from build123d import *

# Parameters (mm, degrees)
F0_R     = 42.5
F0_R_2   = 27.5
F1_DEPTH = 33.5
F2_R     = 100
F2_R_2   = 42.5
F2_R_3   = 27.5
F3_DEPTH = 4
F4_R     = 100
F4_R_2   = 42.5
F4_R_3   = 27.5
F5_DEPTH = 4


# Not quite as in the source:
# - a feature names something its author has since deleted; it is built from what else it names


with BuildPart() as f1:
    # F0 (on Right) → F1 (new body, symmetric)
    with BuildSketch(Plane.YZ):
        Circle(F0_R)
        Circle(F0_R_2, mode=Mode.SUBTRACT)
    extrude(amount=F1_DEPTH, both=True)

    # F2 (on face) → F3 (join)
    with BuildSketch(Plane.YZ.offset(33.5)):
        Circle(F2_R)
        Circle(F2_R_2, mode=Mode.SUBTRACT)
        Circle(F2_R_2)
        Circle(F2_R_3, mode=Mode.SUBTRACT)
    extrude(amount=F3_DEPTH)

    # F4 (on face) → F5 (join)
    with BuildSketch(Plane(origin=(-33.5, 0, 0), x_dir=(0, -1, 0), z_dir=(-1, 0, 0))):
        Circle(F4_R)
        Circle(F4_R_2, mode=Mode.SUBTRACT)
        Circle(F4_R_2)
        Circle(F4_R_3, mode=Mode.SUBTRACT)
    extrude(amount=F5_DEPTH)


solid = f1.part
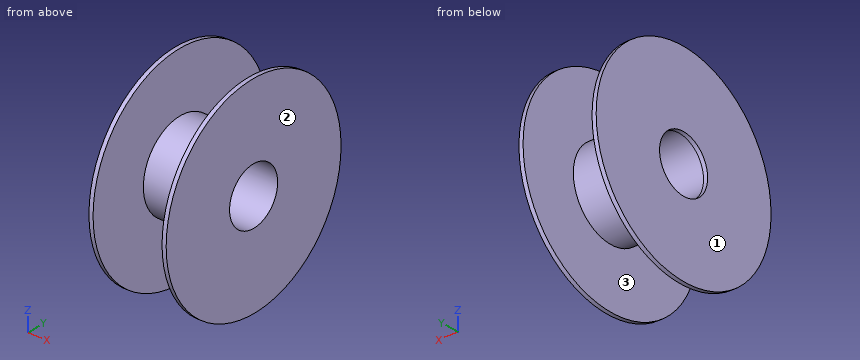
Here's how the part is built. I have some questions about the finished solid (model axes, mm). Face numbers are marked on the shaded views. Round coordinates to 2 decimals unless told otherwise and drop trailing zeros. Write each loop counter-clockwise with the first axis right and the second up, starting at its lowest first coordinate (ties: lowest second). Pieces come first, ordered by that corner, then holes.
1. Suppose I cut it at D-D (x = 2). List the corners of the cut face in (y, z) for me, and give its area (3 significant figures).
2. I need wall thicknesses on L1, parallel to Z at x = -0.5, y = 1.5; L2, parallel to X at y = -35, z = 53.5; L3, parallel to Z at x = -34.5, y = 0. Which ranges of each line are inside material? Lowest first, please.
3. If we mould it in two halves opening along X, with no side actions, what happens to the marked faces 1, 2 and 3? For each: released by +X, released by -X, zero draft, split by the parting line, or undercut.
4. Will this pin go through, and if not, where does the flat tip stop? pin 1 Ø10 at (x, y) = (-13, -7) entering from +Z.
5. Suppose I cut it at C-C (y = -55). List the corners of the cut face in (x, z) for me.
6. Suppose I cut it at A-A (y = 0). List the corners of the cut face in (x, z) for me, and give its area (3 significant figures).
Answer sheet:
1. outline: circle Ø85 at (0, 0); hole circle Ø55 at (0, 0)
1. area: 3,300 mm2
2. L1: z = -42.47 to -27.46, 27.46 to 42.47
2. L2: x = -37.5 to -33.5, 33.5 to 37.5
2. L3: z = -100 to -27.5, 27.5 to 100
3. face 1: released by -X
3. face 2: released by +X
3. face 3: undercut
4. pin 1: stops at z = 42.45
5. outline: (-37.5, -83.52) - (-33.5, -83.52) - (-33.5, 83.52) - (-37.5, 83.52) - close; (33.5, -83.52) - (37.5, -83.52) - (37.5, 83.52) - (33.5, 83.52) - close
6. outline: (-37.5, -100) - (-33.5, -100) - (-33.5, -42.5) - (33.5, -42.5) - (33.5, -100) - (37.5, -100) - (37.5, -27.5) - (-37.5, -27.5) - close; (-37.5, 27.5) - (37.5, 27.5) - (37.5, 100) - (33.5, 100) - (33.5, 42.5) - (-33.5, 42.5) - (-33.5, 100) - (-37.5, 100) - close
6. area: 3,170 mm2
